For this review, take the finished solid that the model builds, in its own axes (mm). Face numbers are marked on the shaded views. A direction names the side the tool comes from. Coordinates: 2 decimals unless noted, no trailing zeros. Order: outer loops, then holes, each group sorted by start corner. A loop starts at its lowest first (then second) coordinate and runs counter-clockwise, first axis right, second up. Notation, with made-up numbers: (-1.5, 85.25) -> (33.5, 85.25) arc R21 ccw to (33.5, 101.25) -> close; hole circle Ø10 at (-16.75, 52.25). An arc over 180 degrees is marked (long way). Answer as a JSON object with one key per item and string values. Group by question number.
1) Add section D-D, the plane y = -1. Write out the cut boundary in (x, z).
2) For pin 1 (4.5 mm diameter, centred on y = 0.5, z = 2, fed in from +X); pin 2 (2.5 mm diameter, centred on y = 0.5, z = 2, fed in from -X); pin 3 (1.5 mm diameter, centred on x = 5.5, y = -12.5, fed in from -Z); pin 4 (12 mm diameter, centred on x = -9, y = -12.5, fed in from -Z), all flat-tipped, find the tip position at first contact; note any pin that passes through.
3) Add section B-B, the plane y = -14. Write out the cut boundary in (x, z), then the cut area to 3 significant figures.
4) Machinability: for the marked faces 4, 5, 6, 7 and 8, which of the approach directions +Z, -Z, +X, -X, +Y, -Y give a long, thin tool a straight path to every point of the face, cutting with its end or side? Answer none if there is none.
5) Draft analysis for pull direction X (two halves, no side actions). For the marked faces 1, 2 and 3, state which applies: +X half, -X half, draft (parallel to the pull), parting line (faces both ways), or undercut.
6) Add section C-C, the plane z = 5.25. Write out the cut boundary in (x, y), then the cut area to 3 significant figures.
7) Add section A-A, the plane x = -7.75. Write out the cut boundary in (y, z), then the cut area to 3 significant figures.
8) Wall thickness on L1, parallel to X at y = -14, z = 6.7; L2, parallel to Y at x = -8.25, z = 0.25; L3, parallel to Y at x = 7.75, z = 6.7: over which ranges is each line inside the solid? List them lowest first.
from build123d import *

# Parameters (mm, degrees)
F0_W      = 24
F0_H      = 5
F0_R      = 1.7
F1_DEPTH  = 7
F2_W      = 24
F2_H      = 7
F3_DEPTH  = 15
F4_R      = 1.6
F5_DEPTH  = 25
F7_DEPTH  = 7
F8_T      = -1
F9_W      = 22
F9_H      = 5.6300974414
F10_DEPTH = 6
F11_W     = 9
F11_H     = 3.6
F12_DEPTH = 1
F13_R     = 1
F14_R     = 1.5
F15_W     = 1
F15_H     = 5
F16_DEPTH = 1


with BuildPart() as f1:
    # F0 (on Top) → F1 (new body)
    with BuildSketch(Plane.XY):
        Rectangle(F0_W, F0_H)
        with Locations((-7, 0)):
            Circle(F0_R, mode=Mode.SUBTRACT)
        with Locations((7, 0)):
            Circle(F0_R, mode=Mode.SUBTRACT)
    extrude(amount=F1_DEPTH)

    # F2 (on face) → F3 (join)
    with BuildSketch(Plane.XZ.offset(2.5)):
        with Locations((0, 3.5)):
            Rectangle(F2_W, F2_H)
    extrude(amount=F3_DEPTH)

    # F4 (on face) → F5 (cut)
    with BuildSketch(Plane(origin=(0, 0, 0), x_dir=(1, 0, 0), z_dir=(0, 0, -1))):
        with Locations((-7.75, 14)):
            Circle(F4_R)
        with Locations((7.75, 14)):
            Circle(F4_R)
    extrude(amount=-F5_DEPTH, mode=Mode.SUBTRACT)

    # F6 (on face) → F7 (cut, through all)
    with BuildSketch(Plane.XY.offset(7)):
        with BuildLine():
            Line((-4.5, 2.5), (-12, 2.5))
            Line((-12, 2.5), (-12, -3.5))
            Line((-12, -3.5), (-6.5, -3.5))
            ThreePointArc((-6.5, -3.5), (-5.0857864376, -2.9142135624), (-4.5, -1.5))
            Line((-4.5, -1.5), (-4.5, 2.5))
        make_face()
        with BuildLine():
            Line((12, -3.5), (12, 2.5))
            Line((12, 2.5), (4.5, 2.5))
            Line((4.5, 2.5), (4.5, -1.5))
            ThreePointArc((4.5, -1.5), (5.0857864376, -2.9142135624), (6.5, -3.5))
            Line((6.5, -3.5), (12, -3.5))
        make_face()
    extrude(amount=-F7_DEPTH, mode=Mode.SUBTRACT)

    # F8
    f8_openings = [f1.faces().sort_by_distance(p)[0] for p in [
        (0, -8.878513, 0),
    ]]
    offset(amount=F8_T, openings=f8_openings)

    # F9 (on face) → F10 (cut, through all)
    with BuildSketch(Plane(origin=(0, 0, 0), x_dir=(1, 0, 0), z_dir=(0, 0, -1))):
        with Locations((0, 13.6849512793)):
            Rectangle(F9_W, F9_H)
    extrude(amount=-F10_DEPTH, mode=Mode.SUBTRACT)

    # F11 (on face) → F12 (cut, through all)
    with BuildSketch(Plane.XZ.offset(17.5)):
        with Locations((0, 2.9600709677)):
            Rectangle(F11_W, F11_H)
    extrude(amount=-F12_DEPTH, mode=Mode.SUBTRACT)

    # F13
    f13_edges = [f1.edges().sort_by_distance(p)[0] for p in [
        (-4.5, -17, 1.160071),
        (4.5, -17, 1.160071),
    ]]
    fillet(f13_edges, radius=F13_R)

    # F14
    f14_edges = [f1.edges().sort_by_distance(p)[0] for p in [
        (12, -17.5, 3.5),
        (11, -16.5, 3),
        (-11, -16.5, 3),
        (-12, -17.5, 3.5),
    ]]
    fillet(f14_edges, radius=F14_R)

    # F15 (on face) → F16 (join)
    with BuildSketch(Plane(origin=(0, 0, 0), x_dir=(1, 0, 0), z_dir=(0, 0, -1))):
        with Locations((11.5, 10)):
            Rectangle(F15_W, F15_H)
        with Locations((-11.5, 10)):
            Rectangle(F15_W, F15_H)
    extrude(amount=F16_DEPTH)


solid = f1.part
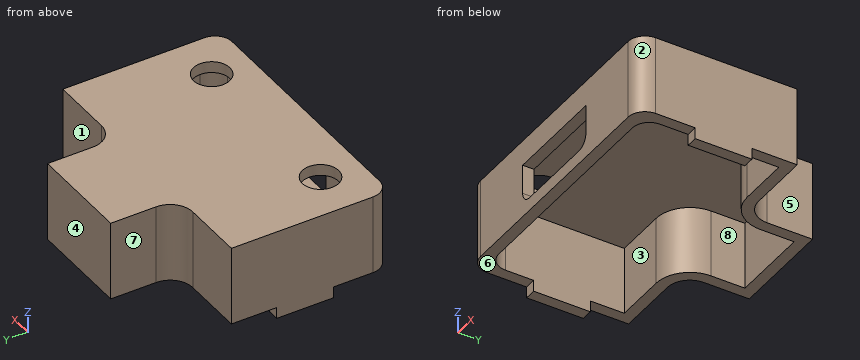
Output values:
{
 "1": {"outline": "(-4.5, 0) -> (-3.5, 0) -> (-3.5, 6) -> (3.5, 6) -> (3.5, 0) -> (4.5, 0) -> (4.5, 7) -> (-4.5, 7) -> close"},
 "2": {"pin 1": "stops at x = 4.52", "pin 2": "stops at x = -4.5", "pin 3": "stops at z = 6", "pin 4": "stops at z = -1"},
 "3": {"outline": "(-12, 0) -> (-11, 0) -> (-11, 6) -> (-9.35, 6) -> (-9.35, 7) -> (-12, 7) -> close; (-6.15, 6) -> (6.15, 6) -> (6.15, 7) -> (-6.15, 7) -> close; (9.35, 6) -> (11, 6) -> (11, 0) -> (12, 0) -> (12, 7) -> (9.35, 7) -> close", "area": "29.6 mm²"},
 "4": {"face 4": "+Z, -Z, +X, -X, +Y", "face 5": "+Z, -Z, +X, +Y", "face 6": "-Z, +X, -X, -Y", "face 7": "+Z, -Z, -X, +Y", "face 8": "-Z"},
 "5": {"face 1": "draft", "face 2": "+X half", "face 3": "undercut"},
 "6": {"outline": "(-12, -16) arc R1.5 ccw to (-10.5, -17.5) -> (10.5, -17.5) arc R1.5 ccw to (12, -16) -> (12, -3.5) -> (6.5, -3.5) arc R2 cw to (4.5, -1.5) -> (4.5, 2.5) -> (-4.5, 2.5) -> (-4.5, -1.5) arc R2 cw to (-6.5, -3.5) -> (-12, -3.5) -> close; hole (-11, -15) arc R1.5 ccw to (-9.5, -16.5) -> (9.5, -16.5) arc R1.5 ccw to (11, -15) -> (11, -4.5) -> (6.5, -4.5) arc R3 cw to (3.5, -1.5) -> (3.5, 1.5) -> (-3.5, 1.5) -> (-3.5, -1.5) arc R3 cw to (-6.5, -4.5) -> (-11, -4.5) -> close", "area": "81.9 mm²"},
 "7": {"outline": "(-17.5, 0) -> (-16.5, 0) -> (-16.5, 6) -> (-15.6, 6) -> (-15.6, 7) -> (-17.5, 7) -> close; (-12.4, 6) -> (-4.5, 6) -> (-4.5, 0) -> (-3.5, 0) -> (-3.5, 7) -> (-12.4, 7) -> close", "area": "22.8 mm²"},
 "8": {"L1": "x = -12 to -9.35, -6.15 to 6.15, 9.35 to 12", "L2": "y = -17.5 to -16.5, -4.5 to -3.5", "L3": "y = -17.5 to -15.6, -12.4 to -3.5"}
}
